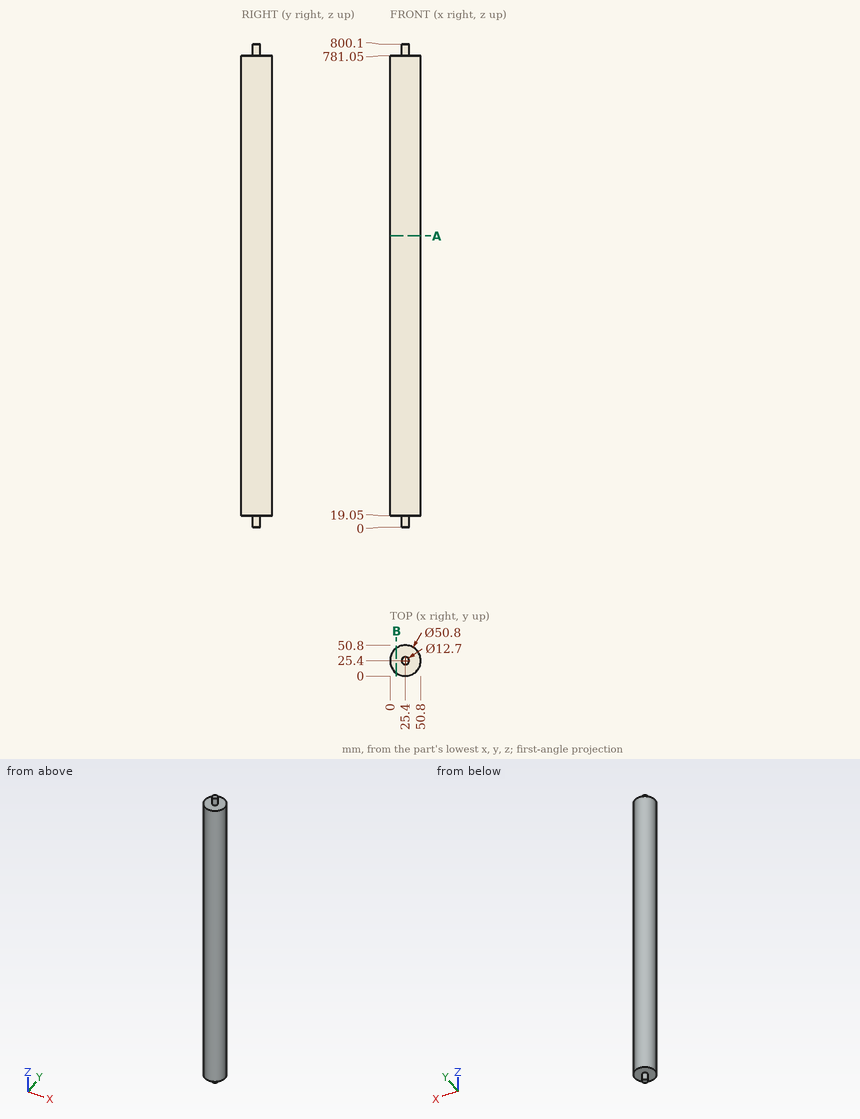
Geometry: see drawing. Coordinates: mm, zero at the bounding-box minimum. Give positions to 0.01 mm unless a question says otherwise; leave off trailing zeros. Order: outer loops, then holes, each group sorted by start corner. A loop starts at its lowest first (then second) coordinate and runs counter-clockwise, first axis right, second up.
Q1. Ray query, probe 1 along Y at (x, z) = (26, 493); probe 2 along Z at (x, y) = (23, 15.5). Return the intervals inside material, ascending.
Checked values:
probe 1: y = 0.01 to 50.79
probe 2: z = 19.05 to 781.05
Q2. Section B-B on x = 10.5. Output: boundary loops of the cut face in (y, z).
Checked values:
outline: (4.83, 19.05) - (45.97, 19.05) - (45.97, 781.05) - (4.83, 781.05) - close
Q3. Contact query for flat-ended pins moving along their axis: pin 1 Ø12 at (x, z) = (43, 609) entering from +Y; pin 2 Ø8 at (y, z) = (45, 656) entering from -X; pin 3 Ø6 at (x, z) = (34, 413) entering from -Y (3 decimals). Output: stop coordinate, or through.
Checked values:
pin 1: stops at y = 48
pin 2: stops at x = 5.36
pin 3: stops at y = 0.625
Q4. Section A-A on z = 482.5. Output: boundary loops of the cut face in (x, y).
Checked values:
outline: circle Ø50.8 at (25.4, 25.4)
